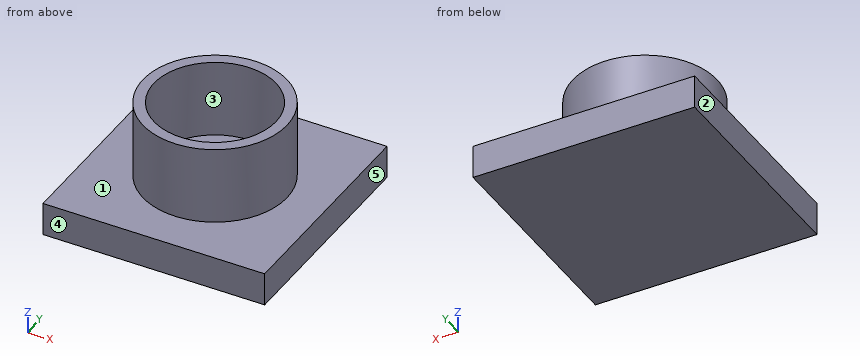
```python
from build123d import *

# Parameters (mm, degrees)
SKETCH_W      = 20
SKETCH_H      = 20
PAD_DEPTH     = 3
SKETCH001_R   = 6.5
SKETCH001_R_2 = 5.5
PAD001_DEPTH  = 10


with BuildPart() as part:
    # Sketch → Pad (new body)
    with BuildSketch(Plane.XY):
        Rectangle(SKETCH_W, SKETCH_H)
    extrude(amount=PAD_DEPTH)

    # Sketch001 → Pad001 (join)
    with BuildSketch(Plane.XY):
        Circle(SKETCH001_R)
        Circle(SKETCH001_R_2, mode=Mode.SUBTRACT)
    extrude(amount=PAD001_DEPTH)


solid = part.part
```
Geometry check sheet. Reference: the model listing, model coordinates, mm. Face numbers are marked on the shaded views. A direction names the side the tool comes from. Coordinates: 2 decimals unless noted, no trailing zeros. Order: outer loops, then holes, each group sorted by start corner. A loop starts at its lowest first (then second) coordinate and runs counter-clockwise, first axis right, second up. Notation, with made-up numbers: (-34, 31) - (4, 31) arc R22 ccw to (4, 39) - close; hole circle Ø5 at (-32.75, -31). An arc over 180 degrees is marked (long way). Answer in a Markdown table with one row per item. Add a question column.
1. Access from +Z, -Z, +X, -X, +Y, -Y to the whole of each face (thin tool, end or side, straight path). Record for the marked faces 1 and 2.
2. Gauge pin test, flat ends, axial feed: pin 1 Ø2 at (x, z) = (-8, 7) entering from +Y; pin 2 Ø3.5 at (x, y) = (2.5, 2.5) entering from +Z; pin 3 Ø4 at (y, z) = (-2.5, 7.5) entering from -X. Record the tip position at first contact, or that the pin passes through.
3. Section check A-A (x = 0). Enter the section's corners in (y, z), plus the area to 3 significant figures.
4. Material ranges on L1, parallel to Y at x = 0, z = 7; L2, parallel to Z at x = 7.75, y = 4, recorded low to high. Write a range as [from, to].
5. Section check C-C (z = 9.25). Enter the section's corners in (x, y).
6. Draft check along X on the marked faces 3, 4 and 5. Enter one of: +X half, -X half, draft (parallel to the pull), parting line (faces both ways), or undercut.
7. Section check D-D (x = 5.75). Enter the section's corners in (y, z).
Data:
| question | item | result |
|---|---|---|
| 1 | face 1 | +Z |
| 1 | face 2 | +Z, -Z, -X, +Y, -Y |
| 2 | pin 1 | passes through |
| 2 | pin 2 | stops at z = 3 |
| 2 | pin 3 | stops at x = -6.48 |
| 3 | outline | (-10, 0) - (10, 0) - (10, 3) - (6.5, 3) - (6.5, 10) - (5.5, 10) - (5.5, 3) - (-5.5, 3) - (-5.5, 10) - (-6.5, 10) - (-6.5, 3) - (-10, 3) - close |
| 3 | area | 74.0 mm² |
| 4 | L1 | y = [-6.5, -5.5], [5.5, 6.5] |
| 4 | L2 | z = [0, 3] |
| 5 | outline | circle Ø13 at (0, 0); hole circle Ø11 at (0, 0) |
| 6 | face 3 | undercut |
| 6 | face 4 | draft |
| 6 | face 5 | +X half |
| 7 | outline | (-10, 0) - (10, 0) - (10, 3) - (3.03, 3) - (3.03, 10) - (-3.03, 10) - (-3.03, 3) - (-10, 3) - close |
